Here's how the part is built. I have some questions about the finished solid (model axes, mm). Coordinates: 2 decimals unless noted, no trailing zeros. Write each loop counter-clockwise with the first axis right and the second up, starting at its lowest first coordinate (ties: lowest second). Pieces come first, ordered by that corner, then holes. Notation, with made-up numbers: (-32, 39.5) -> (10, 39.5) arc R22 ccw to (10, 60.5) -> close; hole circle Ø11 at (-37, -0.5). An arc over 180 degrees is marked (long way). Use a Markdown table: item, result. Add a question column.
Item 1: Imagine slicing it at C-C, the plane z = 28.5. Write out the boundary of the cut face in (x, y).
Item 2: Imagine slicing it at D-D, the plane y = 11. Write out the boundary of the cut face in (x, z).
Item 3: If I drill on line 1 along Y through (x, z) = (-15, 17); line 2 along Z through (x, y) = (-13.5, 1); line 3 along Z through (x, y) = (8.5, 4), over which ranges is the centre line in solid material (lowest first)? Write a range as from..to.
Item 4: Imagine slicing it at A-A, the plane y = -5.5. Write out the boundary of the cut face in (x, z), and give its area (3 significant figures).
Item 5: Will these pins go through, and if not, where does the flat tip stop? pin 1 Ø3 at (y, z) = (8, 20) entering from -X; pin 2 Ø6 at (x, z) = (8, 31.5) entering from +Y; pin 3 Ø12 at (x, y) = (-2.5, 9) entering from -Z.
Item 6: Imagine slicing it at B-B, the plane x = 15. Write out the boundary of the cut face in (y, z), and give its area (3 significant figures).
```python
from build123d import *

# Parameters (mm, degrees)
F5_COUNT = 4
F6_COUNT = 2
F6_ANGLE = 90


with BuildPart() as f2:
    # F0 (on Front) → F2 section 0
    with BuildSketch(Plane.XZ, mode=Mode.PRIVATE) as f2_s0:
        Polygon((-12.204321, 0), (12.204321, 0), (19.747007, 23.213998), (0, 37.561038), (-19.747007, 23.213998), align=None)
    loft([f2_s0.sketch, Vertex(0, 38.1, 16.787151)])

    # F4: F2 across plane


with BuildPart() as f2_1:
    add(f2.part)
    add(f2.part.mirror(Plane.XZ))


with BuildPart() as f5_1:
    # F5: instance of F2
    add(f2_1.part.rotate(Axis((0, 0, 18.392423), (0, 0, 1)), 1 * 360 / F5_COUNT))


with BuildPart() as f5_2:
    # F5: instance of F2
    add(f2_1.part.rotate(Axis((0, 0, 18.392423), (0, 0, 1)), 2 * 360 / F5_COUNT))


with BuildPart() as f5_3:
    # F5: instance of F2
    add(f2_1.part.rotate(Axis((0, 0, 18.392423), (0, 0, 1)), 3 * 360 / F5_COUNT))


with BuildPart() as f6_1:
    # F6: instance of F2
    add(f2_1.part.rotate(Axis((0.121067, 0, 18.392423), (-1, 0, 0)), 1 * F6_ANGLE / (F6_COUNT - 1)))


with BuildPart() as f2_2:
    add(f2_1.part)

    # F7: intersect F5_1, F6_1, F5_2, F5_3
    add(f5_1.part, mode=Mode.INTERSECT)
    add(f6_1.part, mode=Mode.INTERSECT)
    add(f5_2.part, mode=Mode.INTERSECT)
    add(f5_3.part, mode=Mode.INTERSECT)


solid = f2_2.part
```
Ans:
| question | item | result |
|---|---|---|
| 1 | outline | (-12.47, 0) -> (-7.12, -7.12) -> (0, -12.47) -> (7.12, -7.12) -> (12.47, 0) -> (7.12, 7.12) -> (0, 12.47) -> (-7.12, 7.12) -> close |
| 2 | outline | (-11.24, 18.39) -> (-1.08, 4.85) -> (1.08, 4.85) -> (11.24, 18.39) -> (4.83, 26.93) -> (0, 29.57) -> (-4.83, 26.93) -> close |
| 3 | line 1 | y = -5.89..5.89 |
| 3 | line 2 | z = 7.59..27.21 |
| 3 | line 3 | z = 3.75..29.2 |
| 4 | outline | (-15.95, 19.36) -> (-13.84, 12.89) -> (-9.89, 4.36) -> (-5.5, 2.42) -> (5.5, 2.42) -> (9.89, 4.36) -> (13.84, 12.89) -> (15.95, 19.36) -> (13.42, 24.81) -> (5.5, 30.57) -> (0, 33.57) -> (-5.5, 30.57) -> (-13.42, 24.81) -> close |
| 4 | area | 710 mm^2 |
| 5 | pin 1 | stops at x = -15.8 |
| 5 | pin 2 | stops at y = 7.04 |
| 5 | pin 3 | stops at z = 1.32 |
| 6 | outline | (-7.83, 19.77) -> (-4.03, 14.36) -> (1.38, 10.57) -> (7.65, 19.52) -> (5.35, 23.74) -> (1.13, 26.05) -> close |
| 6 | area | 133 mm^2 |
